Geometry check sheet. Reference: the model listing, model coordinates, mm. A direction names the side the tool comes from. Coordinates: 2 decimals unless noted, no trailing zeros. Order: outer loops, then holes, each group sorted by start corner. A loop starts at its lowest first (then second) coordinate and runs counter-clockwise, first axis right, second up. Notation, with made-up numbers: (5.5, 48) - (42.5, 48) arc R19 cw to (42.5, 69) - close; hole circle Ø9 at (11, 15.5). An arc over 180 degrees is marked (long way). Return JSON: item names as keys, results as strings. Group by question number.
Item 1: Section check D-D on x = 17.5. Enter the section's corners in (y, z).
Item 2: Section check A-A on x = 30.25. Enter the section's corners in (y, z), then the cut area to 3 significant figures.
Item 3: Tool access check on faces 5 (the cylindrical face through (27.869, 12.925, 3.521)), 6 (the cylindrical face through (16.11, 3.94, 3.48)). Record the directions out of +Z, -Z, +X, -X, +Y, -Y that give a thin tool (end or side, any length) a straight path to the whole face; none if there is none.
Item 4: Draft check along X on faces 1 (the cylindrical face through (28.04, 42.28, 3.52)), 2 (the cylindrical face through (28.86, 39.19, 0.99)), 3 (the flat face through (0, 27, 2)), 4 (the flat face through (17, 28, 5)). Enter one of: pulls with the +X half, pulls with the -X half, needs draft (parallel to the pull), parting line crosses it, or undercut.
Item 5: Gauge pin test, flat ends, axial feed: pin 1 (2 mm diameter, centred on y = 31.5, z = 0.5, fed in from -X); pin 2 (5.5 mm diameter, centred on x = 4.75, y = 40.25, fed in from +Z); pin 3 (4 mm diameter, centred on x = 17.5, y = 50, fed in from -Z). Record the tip position at first contact, or that the pin passes through.
Item 6: Scan lines: probe 1 along X at (y, z) = (14.75, 1.55); probe 2 along Y at (x, z) = (4.75, 1.3); probe 3 along Y at (x, z) = (17.5, 3.95). Record each from-to range of solid material in increasing order.
Item 7: Section check B-B on z = 4.3. Enter the section's corners in (x, y).
Item 8: Section check C-C on y = 40.25. Enter the section's corners in (x, z).
from build123d import *

# Parameters (mm, degrees)
SKETCH1_W           = 35
SKETCH1_H           = 55
SKETCH1_R           = 1.75
BOSS_EXTRUDE1_DEPTH = 5
SKETCH2_R           = 3
CUT_EXTRUDE1_DEPTH  = 3
CHAMFER1_SIZE       = 2


with BuildPart() as part:
    # Sketch1 → Boss-Extrude1 (new body)
    with BuildSketch(Plane.XY):
        with Locations((17.5, 27.5)):
            Rectangle(SKETCH1_W, SKETCH1_H)
        with Locations((4.75, 40.25)):
            Circle(SKETCH1_R, mode=Mode.SUBTRACT)
        with Locations((30.25, 40.25)):
            Circle(SKETCH1_R, mode=Mode.SUBTRACT)
        with Locations((30.25, 14.75)):
            Circle(SKETCH1_R, mode=Mode.SUBTRACT)
        with Locations((4.75, 14.75)):
            Circle(SKETCH1_R, mode=Mode.SUBTRACT)
        with Locations((17.5, 50)):
            Circle(SKETCH1_R, mode=Mode.SUBTRACT)
        with Locations((17.5, 5)):
            Circle(SKETCH1_R, mode=Mode.SUBTRACT)
    extrude(amount=BOSS_EXTRUDE1_DEPTH)

    # Sketch2 → Cut-Extrude1 (cut)
    with BuildSketch(Plane.XY.offset(5)):
        with Locations((4.75, 40.25)):
            Circle(SKETCH2_R)
        with Locations((30.25, 40.25)):
            Circle(SKETCH2_R)
        with Locations((30.25, 14.75)):
            Circle(SKETCH2_R)
        with Locations((4.75, 14.75)):
            Circle(SKETCH2_R)
    extrude(amount=-CUT_EXTRUDE1_DEPTH, mode=Mode.SUBTRACT)

    # Chamfer1
    chamfer1_edges = [part.edges().sort_by_distance(p)[0] for p in [
        (15.75, 50, 0),
        (15.75, 5, 0),
    ]]
    chamfer(chamfer1_edges, length=CHAMFER1_SIZE)


solid = part.part
Computed:
{
 "1": {"outline": "(0, 0) - (1.25, 0) - (3.25, 2) - (3.25, 5) - (0, 5) - close; (6.75, 2) - (8.75, 0) - (46.25, 0) - (48.25, 2) - (48.25, 5) - (6.75, 5) - close; (51.75, 2) - (53.75, 0) - (55, 0) - (55, 5) - (51.75, 5) - close"},
 "2": {"outline": "(0, 0) - (13, 0) - (13, 2) - (11.75, 2) - (11.75, 5) - (0, 5) - close; (16.5, 0) - (38.5, 0) - (38.5, 2) - (37.25, 2) - (37.25, 5) - (17.75, 5) - (17.75, 2) - (16.5, 2) - close; (42, 0) - (55, 0) - (55, 5) - (43.25, 5) - (43.25, 2) - (42, 2) - close", "area": "225 mm²"},
 "3": {"face 5": "+Z", "face 6": "+Z, -Z"},
 "4": {"face 1": "undercut", "face 2": "undercut", "face 3": "pulls with the -X half", "face 4": "needs draft"},
 "5": {"pin 1": "stops at x = 0", "pin 2": "stops at z = 2", "pin 3": "stops at z = 1.75"},
 "6": {"probe 1": "x = 0 to 3, 6.5 to 28.5, 32 to 35", "probe 2": "y = 0 to 13, 16.5 to 38.5, 42 to 55", "probe 3": "y = 0 to 3.25, 6.75 to 48.25, 51.75 to 55"},
 "7": {"outline": "(0, 0) - (35, 0) - (35, 55) - (0, 55) - close; hole circle Ø6 at (4.75, 14.75); hole circle Ø6 at (4.75, 40.25); hole circle Ø3.5 at (17.5, 5); hole circle Ø3.5 at (17.5, 50); hole circle Ø6 at (30.25, 14.75); hole circle Ø6 at (30.25, 40.25)"},
 "8": {"outline": "(0, 0) - (3, 0) - (3, 2) - (1.75, 2) - (1.75, 5) - (0, 5) - close; (6.5, 0) - (28.5, 0) - (28.5, 2) - (27.25, 2) - (27.25, 5) - (7.75, 5) - (7.75, 2) - (6.5, 2) - close; (32, 0) - (35, 0) - (35, 5) - (33.25, 5) - (33.25, 2) - (32, 2) - close"}
}
